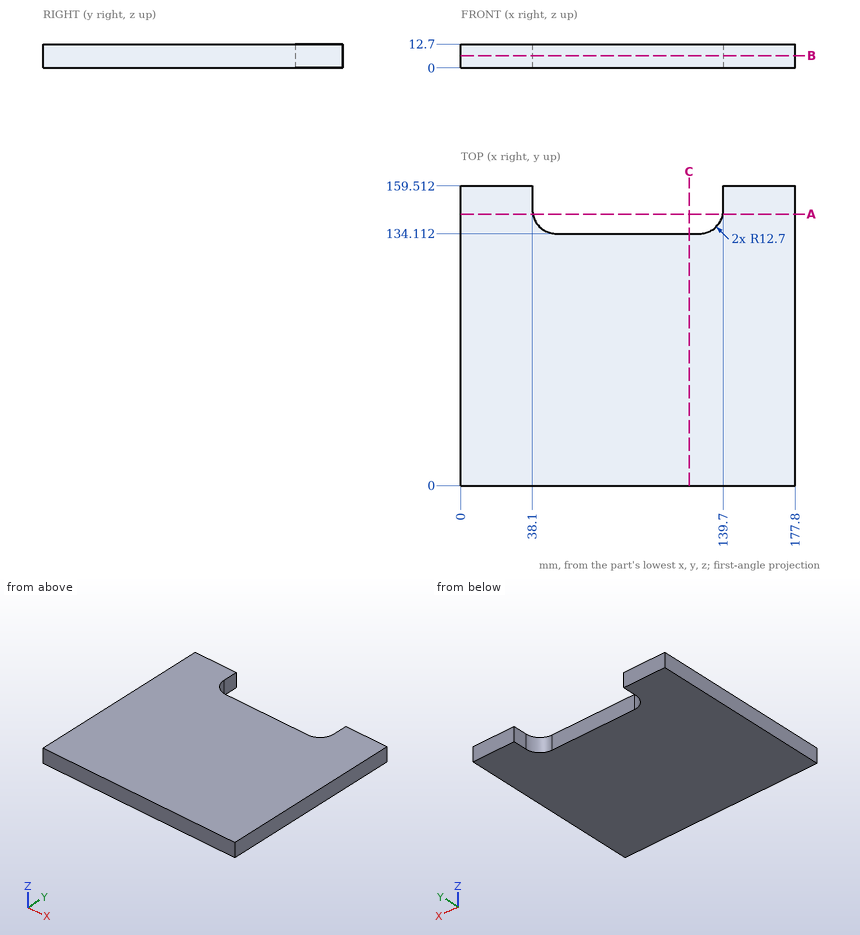
Design review of the part shown in the three views and the two pictorial views. Dimensions are in mm from the part's minimum x, y and z. Coordinates: 2 decimals unless noted, no trailing zeros. Loops run counter-clockwise (first coordinate to the right, second up) from the corner with the lowest first, then second, coordinate; pieces in that order, holes last. Notation, with made-up numbers: M 11.5,-15.75 L 62.5,-15.75 A17 cw 62.5,9.25 Z; hole C -30,-23.75 d9. An arc over 180 degrees is marked long. Put each result on its own line as item: value. Start each with the question number.
Q1. Add section A-A (y = 144.5). Write out the cut boundary in (x, z), and give its area (3 significant figures).
Q2. Wall thickness on line 1 (X direction, y = 152, z = 8.5); line 2 (Y direction, x = 97.5, z = 11.25); line 3 (X direction, y = 139, z = 7.75): over which ranges is each line inside the solid? List them lowest first.
Q3. Add section B-B (z = 6.5). Write out the cut boundary in (x, y).
Q4. Add section C-C (x = 121.5). Write out the cut boundary in (y, z), and give its area (3 significant figures).
Answers:
1. outline: M 0,0 L 38.31,0 L 38.31,12.7 L 0,12.7 Z; M 139.49,0 L 177.8,0 L 177.8,12.7 L 139.49,12.7 Z
1. area: 973 mm^2
2. line 1: x = 0 to 38.1, 139.7 to 177.8
2. line 2: y = 0 to 134.11
2. line 3: x = 0 to 40.79, 137.01 to 177.8
3. outline: M 0,0 L 177.8,0 L 177.8,159.51 L 139.7,159.51 L 139.7,146.81 A12.7 cw 127,134.11 L 50.8,134.11 A12.7 cw 38.1,146.81 L 38.1,159.51 L 0,159.51 Z
4. outline: M 0,0 L 134.11,0 L 134.11,12.7 L 0,12.7 Z
4. area: 1,700 mm^2
